Geometry check sheet. Reference: the model listing, model coordinates, mm. Round coordinates to 2 decimals unless told otherwise and drop trailing zeros. Write each loop counter-clockwise with the first axis right and the second up, starting at its lowest first coordinate (ties: lowest second). Pieces come first, ordered by that corner, then holes.
Item 1: Scan lines: probe 1 along Z at (x, y) = (71, -22.5) (3 decimals); probe 2 along X at (y, z) = (-24.5, -32.5) (3 decimals); probe 3 along Y at (x, z) = (184.5, 92.5). Record each from-to range of solid material in increasing order.
Item 2: Depth check by flat-ended pin: P1, Ø7, axis at x = -45, y = -23.5, coming from the -Z side (3 decimals). Enter the tip coordinate at first touch or a pass-through.
Item 3: Cross-section at B-B (z = 49). Enter the section's corners in (x, y) (3 decimals).
Item 4: Cross-section at A-A (x = 105.5). Enter the section's corners in (y, z) (3 decimals).
from build123d import *

# Parameters (mm, degrees)
F0_W     = 203.2
F0_H     = 558.8
F1_DEPTH = 25.4


with BuildPart() as f1:
    # F0 (on Front) → F1 (new body)
    with BuildSketch(Plane.XZ):
        with Locations((101.6, 0)):
            Rectangle(F0_W, F0_H)
    extrude(amount=F1_DEPTH)

    # F4: sweep along a path in F3
    with BuildLine(Plane.XZ.offset(25.4)) as f4_path:
        Line((0, -238.125), (161.925, -238.125))
        Line((161.925, -238.125), (161.925, 238.125))
        Line((161.925, 238.125), (0, 238.125))
    # F2 (on Right) → F4 (sweep, cut)
    with BuildSketch(Plane.YZ):
        Polygon((-19.05, -263.525), (-19.05, -238.125), (-25.4, -238.125), (-25.4, -279.4), (-19.05, -279.4), (-19.05, -276.225), (-22.225, -273.05), (-22.225, -266.7), align=None)
    sweep(path=f4_path.line, transition=Transition.RIGHT, mode=Mode.SUBTRACT)

    # F5: F1 across plane


with BuildPart() as f1_1:
    add(f1.part)
    add(f1.part.mirror(Plane.YZ))


solid = f1_1.part
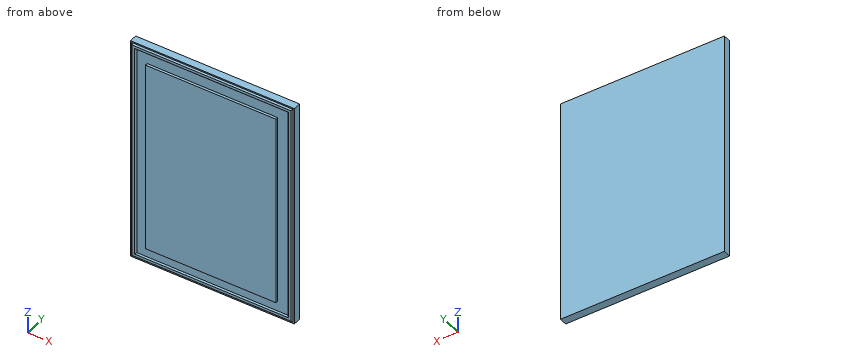
Resolved:
1. probe 1: z = -238.125 to 238.125
1. probe 2: x = -161.925 to 161.925
1. probe 3: y = -19.05 to 0
2. P1: stops at z = -275.275
3. outline: (-203.2, -19.05) - (-200.025, -19.05) - (-196.85, -22.225) - (-190.5, -22.225) - (-187.325, -19.05) - (-161.925, -19.05) - (-161.925, -25.4) - (161.925, -25.4) - (161.925, -19.05) - (187.325, -19.05) - (190.5, -22.225) - (196.85, -22.225) - (200.025, -19.05) - (203.2, -19.05) - (203.2, 0) - (-203.2, 0) - close
4. outline: (-25.4, -238.125) - (-19.05, -238.125) - (-19.05, -263.525) - (-22.225, -266.7) - (-22.225, -273.05) - (-19.05, -276.225) - (-19.05, -279.4) - (0, -279.4) - (0, 279.4) - (-19.05, 279.4) - (-19.05, 276.225) - (-22.225, 273.05) - (-22.225, 266.7) - (-19.05, 263.525) - (-19.05, 238.125) - (-25.4, 238.125) - close
